Work out the finished part from the listing and answer in its coordinate system (mm). A direction names the side the tool comes from. Round coordinates to 2 decimals unless told otherwise and drop trailing zeros. Write each loop counter-clockwise with the first axis right and the second up, starting at its lowest first coordinate (ties: lowest second). Pieces come first, ordered by that corner, then holes. Notation, with made-up numbers: M -40,-3.5 L 18,-3.5 A14 ccw 18,10.5 Z; hole C 87,32.5 d9. An arc over 180 degrees is marked long. One line per item, written item: value. Start each with the question number.
Q1. Given pin 1 Ø1.6 at (y, z) = (-46.5, 1) entering from +X (3 decimals); pin 2 Ø1.5 at (x, z) = (-64, 1.5) entering from -Y; pin 3 Ø1 at (y, z) = (-67.5, 1.5) entering from -X (3 decimals); pin 4 Ø8 at (x, y) = (-16.5, -47.5) entering from -Z, each flat-ended and moving along its own axis, determine where each tip first touches the part or whether it passes through.
Q2. The mould has two halves that part along Y. Classify faces 4 (the flat face through (-44.45, 2, 2)), 5 (the cylindrical face through (24.874, -106.044, 1.565)), 6 (the flat face through (6, 3.175, 2)): released by +Y, released by -Y, zero draft, split by the parting line, or undercut.
Q3. Find section B-B (y = -72.5). Write down the section's boundary in (x, z) (3 decimals), and give its area (3 significant figures).
Q4. Consider probe 1 along X at (y, z) = (-104, 2.75) (3 decimals); probe 2 along X at (y, z) = (-95, 0.5) (3 decimals); probe 3 along Y at (x, z) = (31, 0.4). Determine where each line is inside the solid, lowest interval first.
Q5. A tool of negligible diameter and unlimited length cuts with its end or side. For faces 1 (the flat face through (12.7, 2, 2)), 2 (the flat face through (12.7, -116, 2)), 3 (the flat face through (0, 2, 2)), from which of +Z, -Z, +X, -X, +Y, -Y can it reach the whole face along a straight path? Write none if from no direction.
Q6. Find section C-C (z = 1.5). Count the separate pieces of the cut face and the enclosed holes in it, and give its area (3 significant figures).
Q7. Find section A-A (x = -27). Write down the section's boundary in (y, z) (3 decimals).
Autodesk Inventor part; units mm, degrees
ref_plane "YZ Plane" through (0, 0, 0) normal (1, 0, 0) x (0, 1, 0)
ref_plane "XZ Plane" through (0, 0, 0) normal (0, 1, 0) x (-1, 0, 0)
ref_plane "XY Plane" through (0, 0, 0) normal (0, 0, 1) x (1, 0, 0)
sketch "Sketch1" plane through (0, 0, 0) normal (0, 0, 1) x (1, 0, 0)
  line L0 (34.925, -114.3) -> (12.7, -114.3)
  line L1 (34.925, -92.075) -> (34.925, -114.3)
  line L2 (38.1, -92.075) -> (34.925, -92.075)
  line L3 (38.1, -79.375) -> (38.1, -92.075)
  line L4 (34.925, -79.375) -> (38.1, -79.375)
  line L5 (34.925, -34.925) -> (34.925, -79.375)
  line L6 (38.1, -34.925) -> (34.925, -34.925)
  line L7 (38.1, -22.225) -> (38.1, -34.925)
  line L8 (34.925, -22.225) -> (38.1, -22.225)
  line L9 (34.925, 0) -> (34.925, -22.225)
  line L10 (12.7, 0) -> (34.925, 0)
  line L11 (12.7, 3.175) -> (12.7, 0)
  line L12 (0, 3.175) -> (12.7, 3.175)
  line L13 (0, 0) -> (0, 3.175)
  line L14 (-44.45, 0) -> (0, 0)
  line L15 (-44.45, 3.175) -> (-44.45, 0)
  line L16 (-57.15, 3.175) -> (-44.45, 3.175)
  line L17 (-57.15, 0) -> (-57.15, 3.175)
  line L18 (-79.375, 0) -> (-57.15, 0)
  line L19 (-79.375, -22.225) -> (-79.375, 0)
  line L20 (-82.55, -22.225) -> (-79.375, -22.225)
  line L21 (-82.55, -34.925) -> (-82.55, -22.225)
  line L22 (-79.375, -34.925) -> (-82.55, -34.925)
  line L23 (-79.375, -79.375) -> (-79.375, -34.925)
  line L24 (-82.55, -79.375) -> (-79.375, -79.375)
  line L25 (-82.55, -92.075) -> (-82.55, -79.375)
  line L26 (-79.375, -92.075) -> (-82.55, -92.075)
  line L27 (-79.375, -114.3) -> (-79.375, -92.075)
  line L28 (-57.15, -114.3) -> (-79.375, -114.3)
  line L29 (-57.15, -117.475) -> (-57.15, -114.3)
  line L30 (-44.45, -117.475) -> (-57.15, -117.475)
  line L31 (-44.45, -114.3) -> (-44.45, -117.475)
  line L32 (0, -114.3) -> (-44.45, -114.3)
  line L33 (0, -117.475) -> (0, -114.3)
  line L34 (12.7, -117.475) -> (0, -117.475)
  line L35 (12.7, -114.3) -> (12.7, -117.475)
  circle A0 centre (-69.5325, -9.8425) radius 1.6
  circle A1 centre (25.0825, -9.8425) radius 1.6
  circle A2 centre (25.0825, -104.4575) radius 1.6
  circle A3 centre (-69.5325, -104.4575) radius 1.6
extrude "Extrusion1" add sketch "Sketch1" along normal blind 3.175
properties part number "Back" material "ABS Plastic"
The answers:
1. pin 1: x = 34.925
1. pin 2: y = -114.3
1. pin 3: x = -79.375
1. pin 4: z = 0
2. face 4: zero draft
2. face 5: undercut
2. face 6: released by +Y
3. outline: M -79.375,0 L 34.925,0 L 34.925,3.175 L -79.375,3.175 Z
3. area: 363 mm2
4. probe 1: -79.375 to -71.066, -67.999 to 23.549, 26.616 to 34.925
4. probe 2: -79.375 to 34.925
4. probe 3: -114.3 to 0
5. face 1: +Z, -Z, +X, +Y
5. face 2: +Z, -Z, +X, -Y
5. face 3: +Z, -Z, +Y
6. separate pieces: 1
6. enclosed holes: 4
6. area: 13,400 mm2
7. outline: M -114.3,0 L 0,0 L 0,3.175 L -114.3,3.175 Z
